```python
from build123d import *

# Parameters (mm, degrees)
SKETCH_1_W          = 59
SKETCH_1_H          = 3
EXTRUDE_1_DEPTH     = 34
SKETCH_2_W          = 3
SKETCH_2_H          = 48
EXTRUDE_2_DEPTH     = 22
SKETCH_3_W          = 43
SKETCH_3_H          = 3
EXTRUDE_3_DEPTH     = 22
SKETCH_4_W          = 48
SKETCH_4_H          = 4.064402022
CUT_EXTRUDE_1_DEPTH = 89


with BuildPart() as part:
    # 草图1 → 凸台-拉伸1 (new body)
    with BuildSketch(Plane(origin=(0, 0, 0), x_dir=(1, 0, 0), z_dir=(0, 1, 0))):
        with Locations((29.5, -1.5)):
            Rectangle(SKETCH_1_W, SKETCH_1_H)
    extrude(amount=EXTRUDE_1_DEPTH)

    # 草图2 → 凸台-拉伸2 (add)
    with BuildSketch(Plane(origin=(0, 34, 0), x_dir=(1, 0, 0), z_dir=(0, 1, 0))):
        with Locations((-1.5, 21)):
            Rectangle(SKETCH_2_W, SKETCH_2_H)
    extrude(amount=-EXTRUDE_2_DEPTH)

    # 草图3 → 凸台-拉伸3 (add)
    with BuildSketch(Plane(origin=(0, 34, 0), x_dir=(1, 0, 0), z_dir=(0, 1, 0))):
        with Locations((18.5, 46.5)):
            Rectangle(SKETCH_3_W, SKETCH_3_H)
    extrude(amount=-EXTRUDE_3_DEPTH)

    # 草图4 → 切除-拉伸1 (cut)
    with BuildSketch(Plane(origin=(40, 0, 0), x_dir=(0, 0, -1), z_dir=(1, 0, 0))):
        with Locations((24, 31.967798989)):
            Rectangle(SKETCH_4_W, SKETCH_4_H)
    extrude(amount=-CUT_EXTRUDE_1_DEPTH, mode=Mode.SUBTRACT)


solid = part.part
```
Source: CAD feature listing. Evaluate the final solid. Frame: model axes, mm. A direction names the side the tool comes from. Round coordinates to 2 decimals unless told otherwise and drop trailing zeros. Loops run counter-clockwise (first coordinate to the right, second up) from the corner with the lowest first, then second, coordinate; pieces in that order, holes last.
(1) Access query for faces 5 (the flat face through (40, 21, -46)), 6 (the flat face through (-1, 29.936, -35)), 7 (the flat face through (0, 6, 2)), 8 (the flat face through (0, 21, -22)), 9 (the flat face through (29, 0, 1)). Directions: +Z, -Z, +X, -X, +Y, -Y. A direction counts if a zero-diameter tool reaches every point of the face in a straight line with its end or side. Return the directions, or none.
From the geometry:
face 5: -Z, +X, +Y, -Y
face 6: -Z, +X, -X, +Y
face 7: +Z, -Z, -X, -Y
face 8: +X, +Y, -Y
face 9: +Z, -Z, +X, -X, -Y
(2) Section query B-B (y = 27). Output: boundary loops of the cut face in (x, z), and give its area (3 significant figures).
From the geometry:
outline: (-3, -48) - (40, -48) - (40, -45) - (0, -45) - (0, 0) - (59, 0) - (59, 3) - (-3, 3) - close
area: 450 mm2
(3) Pull-direction query (Z, two-part tool) for faces 1 (the flat face through (28, 17, 3)), 2 (the flat face through (28, 17, 0)), 3 (the flat face through (-3, 21, -22)), 4 (the flat face through (20, 21, -45)); classes: +Z half, -Z half, draft (parallel to the pull), parting line (faces both ways), or undercut.
From the geometry:
face 1: +Z half
face 2: undercut
face 3: draft
face 4: undercut
(4) Contact query for flat-ended pins moving along their axis: pin 1 Ø1.5 at (y, z) = (8, 1) entering from -X; pin 2 Ø2 at (y, z) = (13.5, -33.5) entering from +X; pin 3 Ø2.5 at (y, z) = (22, -46.5) entering from +X. Output: stop coordinate, or through.
From the geometry:
pin 1: stops at x = 0
pin 2: stops at x = 0
pin 3: stops at x = 40
(5) Section query C-C (z = -19). Output: boundary loops of the cut face in (x, y), and give its area (3 significant figures).
From the geometry:
outline: (-3, 12) - (0, 12) - (0, 29.94) - (-3, 29.94) - close
area: 53.8 mm2
(6) Section query A-A (x = 28.5). Output: boundary loops of the cut face in (y, z), and give its area (3 significant figures).
From the geometry:
outline: (0, 0) - (34, 0) - (34, 3) - (0, 3) - close; (12, -48) - (29.94, -48) - (29.94, -45) - (12, -45) - close
area: 156 mm2
(7) Section query D-D (x = 52). Output: boundary loops of the cut face in (y, z), and give its area (3 significant figures).
From the geometry:
outline: (0, 0) - (34, 0) - (34, 3) - (0, 3) - close
area: 102 mm2
(8) Material intervals for probe 1 along Z at (x, y) = (3.5, 20); probe 2 along X at (y, z) = (27.5, -3); probe 3 along Z at (x, y) = (40.5, 29.5), sorted ascending.
From the geometry:
probe 1: z = -48 to -45, 0 to 3
probe 2: x = -3 to 0
probe 3: z = 0 to 3
